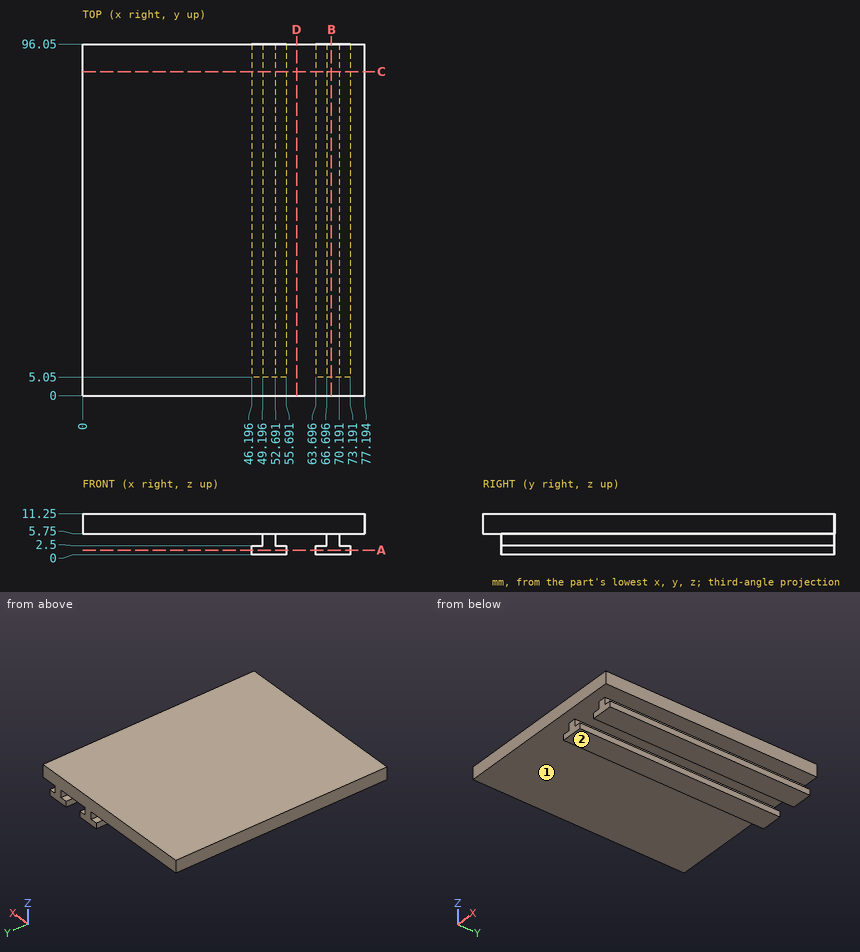
Study the drawing (mm; zero at the part's minimum x, y, z) and answer. Round coordinates to 2 decimals unless told otherwise and drop trailing zeros. Write each loop counter-clockwise with the first axis right and the second up, starting at its lowest first coordinate (ties: lowest second). Pieces come first, ordered by that corner, then holes.
1) A cutting plane is placed at D-D (x = 58.5). Give the vertices of the cut face in (y, z), plus the area to 3 significant figures.
2) Straight lines are drawn through the part: line 1 (Z direction, x = 55.5, y = 27.5); line 2 (X direction, y = 18, z = 2.25); line 3 (X direction, y = 65, z = 4). For each, find the intervals that lie inside material, in ascending order.
3) A cutting plane is placed at B-B (x = 68). Give the vertices of the cut face in (y, z), plus the area to 3 significant figures.
4) A cutting plane is placed at A-A (z = 1.25). Give the vertices of the cut face in (x, y).
5) Given pin 1 Ø1 at (y, z) = (40.5, 4.5) entering from -X; pin 2 Ø12 at (x, y) = (10.5, 59) entering from -Z; pin 3 Ø3.5 at (y, z) = (32.5, 3.5) entering from +X, each flat-ended and moving along its own axis, determine where each tip first touches the part or whether it passes through.
6) A cutting plane is placed at C-C (y = 88.5). Give the vertices of the cut face in (x, z), plus the area to 3 significant figures.
7) The mould has two halves that part along X. Classify the marked faces 1 and 2: pulls with the +X half, pulls with the -X half, needs draft (parallel to the pull), parting line crosses it, or undercut.
Completed:
1. outline: (0, 5.75) - (96.05, 5.75) - (96.05, 11.25) - (0, 11.25) - close
1. area: 528 mm2
2. line 1: z = 0 to 2.5, 5.75 to 11.25
2. line 2: x = 46.2 to 55.69, 63.7 to 73.19
2. line 3: x = 49.2 to 52.69, 66.7 to 70.19
3. outline: (0, 5.75) - (5.05, 5.75) - (5.05, 0) - (96.05, 0) - (96.05, 11.25) - (0, 11.25) - close
3. area: 1,050 mm2
4. outline: (46.2, 5.05) - (55.69, 5.05) - (55.69, 96.05) - (46.2, 96.05) - close; (63.7, 5.05) - (73.19, 5.05) - (73.19, 96.05) - (63.7, 96.05) - close
5. pin 1: stops at x = 49.2
5. pin 2: stops at z = 5.75
5. pin 3: stops at x = 73.19
6. outline: (0, 5.75) - (49.2, 5.75) - (49.2, 2.5) - (46.2, 2.5) - (46.2, 0) - (55.69, 0) - (55.69, 2.5) - (52.69, 2.5) - (52.69, 5.75) - (66.7, 5.75) - (66.7, 2.5) - (63.7, 2.5) - (63.7, 0) - (73.19, 0) - (73.19, 2.5) - (70.19, 2.5) - (70.19, 5.75) - (77.19, 5.75) - (77.19, 11.25) - (0, 11.25) - close
6. area: 495 mm2
7. face 1: undercut
7. face 2: needs draft
